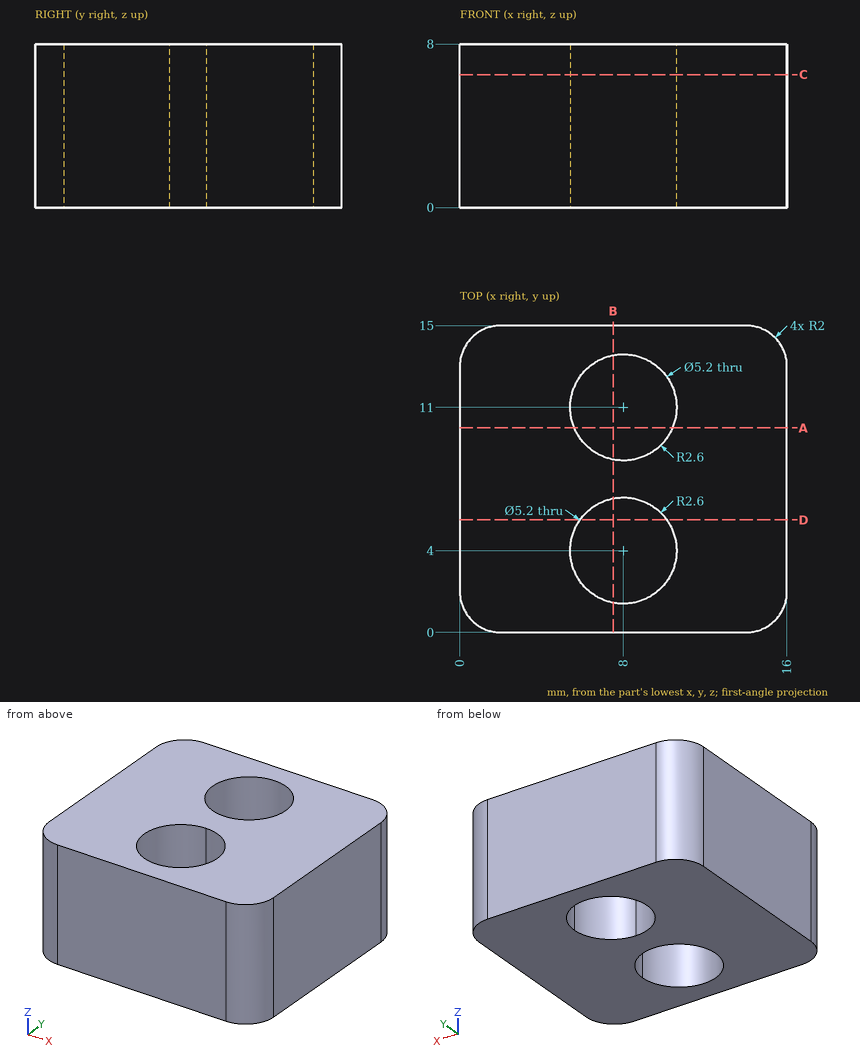
Part print with two shaded views. Sizes in mm from the minimum x, y, z corner. Coordinates: 2 decimals unless noted, no trailing zeros. Write each loop counter-clockwise with the first axis right and the second up, starting at its lowest first coordinate (ties: lowest second). Pieces come first, ordered by that corner, then holes. Notation, with made-up numbers: (73.5, 17) - (101.5, 17) arc R16 cw to (101.5, 34) - close; hole circle Ø2 at (80.25, -1.75). An arc over 180 degrees is marked (long way). Use a Markdown table: item, result. Add a question column.
Item 1: Band-saw the part on D-D, the plane y = 5.5. Write the cut outline in (x, z), and give its area (3 significant figures).
Item 2: Drill centre lines: line 1 along Y through (x, z) = (8, 2); line 2 along Y through (x, z) = (6.25, 5.5); line 3 along X through (y, z) = (3.75, 3.75). Where is each one in solid material? Low to high.
Item 3: Drop a flat-ended pin along its axis: pin 1 (8.5 mm diameter, centred on x = 8, y = 11, fed in from -Z). Give the stop position or say it passes through.
Item 4: Band-saw the part on A-A, the plane y = 10. Write the cut outline in (x, z).
Item 5: Band-saw the part on C-C, the plane z = 6.5. Write the cut outline in (x, y), and give its area (3 significant figures).
Item 6: Band-saw the part on B-B, the plane x = 7.5. Write the cut outline in (y, z).
A:
| question | item | result |
|---|---|---|
| 1 | outline | (0, 0) - (5.88, 0) - (5.88, 8) - (0, 8) - close; (10.12, 0) - (16, 0) - (16, 8) - (10.12, 8) - close |
| 1 | area | 94.0 mm² |
| 2 | line 1 | y = 0 to 1.4, 6.6 to 8.4, 13.6 to 15 |
| 2 | line 2 | y = 0 to 2.08, 5.92 to 9.08, 12.92 to 15 |
| 2 | line 3 | x = 0 to 5.41, 10.59 to 16 |
| 3 | pin 1 | stops at z = 0 |
| 4 | outline | (0, 0) - (5.6, 0) - (5.6, 8) - (0, 8) - close; (10.4, 0) - (16, 0) - (16, 8) - (10.4, 8) - close |
| 5 | outline | (0, 2) arc R2 ccw to (2, 0) - (14, 0) arc R2 ccw to (16, 2) - (16, 13) arc R2 ccw to (14, 15) - (2, 15) arc R2 ccw to (0, 13) - close; hole circle Ø5.2 at (8, 4); hole circle Ø5.2 at (8, 11) |
| 5 | area | 194 mm² |
| 6 | outline | (0, 0) - (1.45, 0) - (1.45, 8) - (0, 8) - close; (6.55, 0) - (8.45, 0) - (8.45, 8) - (6.55, 8) - close; (13.55, 0) - (15, 0) - (15, 8) - (13.55, 8) - close |
